For this review, take the finished solid that the model builds, in its own axes (mm). Round coordinates to 2 decimals unless told otherwise and drop trailing zeros. Write each loop counter-clockwise with the first axis right and the second up, starting at its lowest first coordinate (ties: lowest second). Pieces come first, ordered by that corner, then holes.
from build123d import *

# Parameters (mm, degrees)
EXTRUDE_1_DEPTH = 4
FILLET_1_R      = 1


with BuildPart() as part:
    # 草图1 → 凸台-拉伸1 (new body)
    with BuildSketch(Plane(origin=(0, 0, 0), x_dir=(1, 0, 0), z_dir=(0, 1, 0))):
        with BuildLine():
            Line((-5.928068954, -6.449296909), (-4.820160255, -3.746554363))
            ThreePointArc((-4.820160255, -3.746554363), (4.093177489, 3.01181264), (13.350341007, 9.290987577))
            Line((13.350341007, 9.290987577), (22.871021424, 11.851023114))
            Line((22.871021424, 11.851023114), (23.289072647, 10.296305596))
            Line((23.289072647, 10.296305596), (13.350341007, 7.623859397))
            ThreePointArc((13.350341007, 7.623859397), (3.511743095, 0.860423855), (-5.928068954, -6.449296909))
        make_face()
    extrude(amount=EXTRUDE_1_DEPTH)

    # 圆角1
    # the kernel refuses this fillet: 1 mm, written as the material it takes off along each edge
    with BuildSketch(Plane(origin=(127.771889532, 4, 169.359958319), x_dir=(-0.6341416592780885, 0, -0.7732168880514914), z_dir=(-0.7732168880514914, 0, 0.6341416592780885))) as fillet_1_piece_1:
        with BuildLine():
            CenterArc((212.151953176 - FILLET_1_R, FILLET_1_R), FILLET_1_R, 270, 90)
            Line((212.151953176 - FILLET_1_R, 0), (212.151953176, 0))
            Line((212.151953176, 0), (212.151953176, FILLET_1_R))
        make_face()
    revolve(axis=Axis((127.771889532, 4, 169.359958319), (0, -1, 0)), revolution_arc=7.865584332, mode=Mode.SUBTRACT)
    # the kernel refuses this fillet: 1 mm, written as the material it takes off along each edge
    with BuildSketch(Plane(origin=(12.521058721, 4, -9.06800014), x_dir=(0.2596684924125265, 0, 0.9656978171499642), z_dir=(0.9656978171499642, 0, -0.2596684924125265))) as fillet_1_2_piece_1:
        with BuildLine():
            CenterArc((FILLET_1_R, FILLET_1_R), FILLET_1_R, 180, 90)
            Line((0, FILLET_1_R), (0, 0))
            Line((0, 0), (FILLET_1_R, 0))
        make_face()
    extrude(amount=13.21759977, mode=Mode.SUBTRACT)
    # the kernel refuses this fillet: 1 mm, written as the material it takes off along each edge
    with BuildSketch(Plane(origin=(25.70331719, 4, -10.945476827), x_dir=(-0.25966849241252477, 0, -0.9656978171499647), z_dir=(-0.9656978171499647, 0, 0.25966849241252477))) as fillet_1_3_piece_1_section:
        with BuildLine():
            CenterArc((FILLET_1_R, FILLET_1_R), FILLET_1_R, 180, 90)
            Line((0, FILLET_1_R), (0, 0))
            Line((0, 0), (FILLET_1_R, 0))
        make_face()
    fillet_1_3_piece_1 = extrude(amount=15.291761526, mode=Mode.PRIVATE)
    fillet_1_3_piece_1 = fillet_1_3_piece_1 & Plane(origin=(127.771889532, 4, 169.359958319), x_dir=(-0.5429254971555654, 0, -0.8397808669756547), z_dir=(0, -1, 0)) * Cylinder(210.75, 35, mode=Mode.PRIVATE)
    add(fillet_1_3_piece_1, mode=Mode.SUBTRACT)
    # the kernel refuses this fillet: 1 mm, written as the material it takes off along each edge
    with BuildSketch(Plane(origin=(127.771889532, 4, 169.359958319), x_dir=(-0.6435256080636699, 0, -0.765424582677016), z_dir=(-0.765424582677016, 0, 0.6435256080636699))) as fillet_1_4_piece_1_section:
        with BuildLine():
            CenterArc((210.75 + FILLET_1_R, FILLET_1_R), FILLET_1_R, 180, 90)
            Line((210.75 + FILLET_1_R, 0), (210.75, 0))
            Line((210.75, 0), (210.75, FILLET_1_R))
        make_face()
    fillet_1_4_piece_1 = revolve(axis=Axis((127.771889532, 4, 169.359958319), (0, -1, 0)), revolution_arc=8.877330019, mode=Mode.PRIVATE)
    fillet_1_4_piece_1 = fillet_1_4_piece_1 - Plane(origin=(75.416344667, 3, -25.348436689), x_dir=(0, 1, 0), z_dir=(0.9656978171499647, 0, -0.25966849241252477)) * Cylinder(1, 848, mode=Mode.PRIVATE)
    add(fillet_1_4_piece_1, mode=Mode.SUBTRACT)


solid = part.part
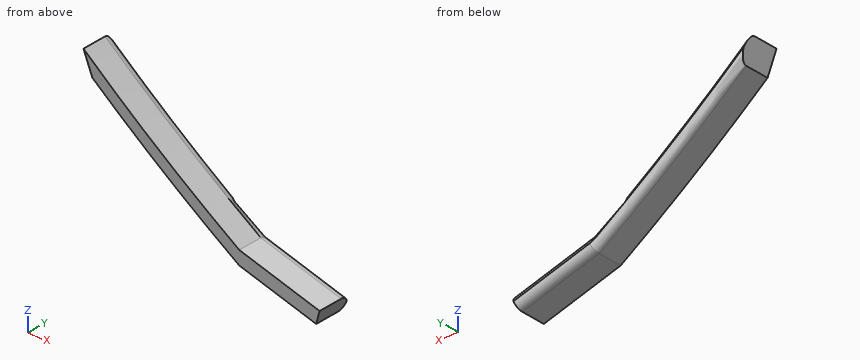
(1) We need section A-A, the plane y = 2.4. Give the boundary of the cut face in (x, z), and give its area (3 significant figures).
Geometry check:
outline: (-5.93, 6.45) - (-4.82, 3.75) arc R212.15 ccw to (13.35, -9.29) - (22.87, -11.85) - (23.29, -10.3) - (13.35, -7.62) arc R210.75 cw to start
area: 48.6 mm2
(2) For pin 1 Ø1 at (x, y) = (5.5, 2.5) entering from +Z; pin 2 Ø2 at (y, z) = (2.5, -6) entering from +X; pin 3 Ø6 at (x, z) = (0.5, -7.5) entering from -Y; pin 4 Ø1.5 at (x, y) = (19, 1) entering from +Z, all flat-tipped, find the tip position at first contact; note any pin that passes through.
Geometry check:
pin 1: stops at z = -1.94
pin 2: stops at x = 12.39
pin 3: passes through
pin 4: stops at z = -8.94
(3) For line 1 along X through (y, z) = (2.2, -7.5); line 2 along Z through (x, y) = (19, 2.6); line 3 along Z through (x, y) = (-3.75, 3.5), list the stretches that pass through material, from the lowest coordinate up.
Geometry check:
line 1: x = 10.6 to 13.16
line 2: z = -10.81 to -9.14
line 3: z = 3.07 to 4.51
